Design review of the part built by this model. Coordinates are the model's own, in mm. A direction names the side the tool comes from. Round coordinates to 2 decimals unless told otherwise and drop trailing zeros. Loops run counter-clockwise (first coordinate to the right, second up) from the corner with the lowest first, then second, coordinate; pieces in that order, holes last. Notation, with made-up numbers: (24.5, -16.75) - (29.5, -16.75) arc R22 cw to (29.5, 14.25) - close; hole circle Ø4 at (-24, -19). An arc over 180 degrees is marked (long way). Return JSON: item names as keys, results as strings. Group by question number.
(1) We need section C-C, the plane z = 2.05. Write out the cut boundary in (x, y).
(2) We need section B-B, the plane y = -4. Write out the cut boundary in (x, z).
(3) Clearance check with flat-ended pins moving along their axes: pin 1 (1.5 mm diameter, centred on x = 6.5, y = 3.5, fed in from -Z); pin 2 (1.4 mm diameter, centred on x = 0, y = -8, fed in from +Z); pin 3 (1 mm diameter, centred on x = -1, z = 2.5, fed in from -Y). State where each tip first meets the part, or that it passes through.
(4) Wall thickness on L1, parallel to Y at x = 0, z = 2.85; L2, parallel to X at y = 3, z = 1.2; L3, parallel to Z at x = -6, y = 3.75: over which ranges is each line inside the solid? List them lowest first. Write a range as [from, to].
(5) For faces 1 (the cylindrical face through (6.265, 3.392, 2.24)), 2 (the cylindrical face through (-7.62, -5.33, 0.74)), list the 3-axis set-ups (+Z, -Z, +X, -X, +Y, -Y) from which the entire face can be reached by the end or side of a thin tool; tool diameter is ignored.
(6) We need section A-A, the plane x = 0. Write out the cut boundary in (y, z), and give its area (3 significant figures).
(7) We need section D-D, the plane y = -8. Write out the cut boundary in (x, z), and give its area (3 significant figures).
(8) The part is to be moulded in two halves that separate along X. For faces 3 (the flat face through (-8, 4, 1.5)), 4 (the flat face through (0, 0, 0)), 5 (the cylindrical face through (-10.316, -7.91, 1.479)), say which applies: pulls with the +X half, pulls with the -X half, needs draft (parallel to the pull), parting line crosses it, or undercut.
from build123d import *

# Parameters (mm, degrees)
SKETCH_1_R               = 13
EXTRUDE_1_DEPTH          = 3
SKETCH_2_R               = 0.9
CUT_EXTRUDE_1_DEPTH      = 19.62793601
SKETCH_2_3_R             = 1.5
CUT_EXTRUDE_2_DEPTH      = 1.5
PATTERN_CIRCULAR_1_COUNT = 6


with BuildPart() as part:
    # Sketch 1 → Extrude 1 (new body)
    with BuildSketch(Plane.XY):
        Circle(SKETCH_1_R)
    extrude(amount=EXTRUDE_1_DEPTH)

    # Sketch 2 → Cut-Extrude 1 (cut, through all)
    with BuildSketch(Plane(origin=(0, 0, 0), x_dir=(-1, 0, 0), z_dir=(0, 0, -1))):
        with Locations((0, 8)):
            Circle(SKETCH_2_R)
    cut_extrude_1 = extrude(amount=-CUT_EXTRUDE_1_DEPTH, mode=Mode.SUBTRACT)

    # Sketch 2_3 → Cut-Extrude 2 (cut)
    with BuildSketch(Plane(origin=(0, 0, 0), x_dir=(-1, 0, 0), z_dir=(0, 0, -1))):
        with Locations((0, 8)):
            Circle(SKETCH_2_3_R)
    cut_extrude_2 = extrude(amount=-CUT_EXTRUDE_2_DEPTH, mode=Mode.SUBTRACT)

    # Pattern Circular 1: Cut-Extrude 1, Cut-Extrude 2 ×6 about axis
    pattern_circular_1_axis = Axis((0, 0, 0), (0, 0, 1))
    add([cut_extrude_1.rotate(pattern_circular_1_axis, i * 360 / PATTERN_CIRCULAR_1_COUNT) for i in range(1, PATTERN_CIRCULAR_1_COUNT)], mode=Mode.SUBTRACT)
    add([cut_extrude_2.rotate(pattern_circular_1_axis, i * 360 / PATTERN_CIRCULAR_1_COUNT) for i in range(1, PATTERN_CIRCULAR_1_COUNT)], mode=Mode.SUBTRACT)


solid = part.part
Solutions:
{
 "1": {"outline": "circle Ø26 at (0, 0); hole circle Ø1.8 at (-6.93, -4); hole circle Ø1.8 at (-6.93, 4); hole circle Ø1.8 at (0, -8); hole circle Ø1.8 at (0, 8); hole circle Ø1.8 at (6.93, -4); hole circle Ø1.8 at (6.93, 4)"},
 "2": {"outline": "(-12.37, 0) - (-8.43, 0) - (-8.43, 1.5) - (-7.83, 1.5) - (-7.83, 3) - (-12.37, 3) - close; (-6.03, 1.5) - (-5.43, 1.5) - (-5.43, 0) - (5.43, 0) - (5.43, 1.5) - (6.03, 1.5) - (6.03, 3) - (-6.03, 3) - close; (7.83, 1.5) - (8.43, 1.5) - (8.43, 0) - (12.37, 0) - (12.37, 3) - (7.83, 3) - close"},
 "3": {"pin 1": "z = 1.5", "pin 2": "through", "pin 3": "y = -12.99"},
 "4": {"L1": "[-13, -8.9], [-7.1, 7.1], [8.9, 13]", "L2": "[-12.65, -8.05], [-5.81, 5.81], [8.05, 12.65]", "L3": "[1.5, 3]"},
 "5": {"face 1": "+Z, -Z", "face 2": "-Z"},
 "6": {"outline": "(-13, 0) - (-9.5, 0) - (-9.5, 1.5) - (-8.9, 1.5) - (-8.9, 3) - (-13, 3) - close; (-7.1, 1.5) - (-6.5, 1.5) - (-6.5, 0) - (6.5, 0) - (6.5, 1.5) - (7.1, 1.5) - (7.1, 3) - (-7.1, 3) - close; (8.9, 1.5) - (9.5, 1.5) - (9.5, 0) - (13, 0) - (13, 3) - (8.9, 3) - close", "area": "63.6 mm^2"},
 "7": {"outline": "(-10.25, 0) - (-1.5, 0) - (-1.5, 1.5) - (-0.9, 1.5) - (-0.9, 3) - (-10.25, 3) - close; (0.9, 1.5) - (1.5, 1.5) - (1.5, 0) - (10.25, 0) - (10.25, 3) - (0.9, 3) - close", "area": "54.3 mm^2"},
 "8": {"face 3": "undercut", "face 4": "needs draft", "face 5": "parting line crosses it"}
}
